Build history of the part. All positions in model axes, mm. A direction names the side the tool comes from. Round coordinates to 2 decimals unless told otherwise and drop trailing zeros. Loops run counter-clockwise (first coordinate to the right, second up) from the corner with the lowest first, then second, coordinate; pieces in that order, holes last. Notation, with made-up numbers: M 71.5,4 L 96.5,4 A9 ccw 96.5,17 Z; hole C 13.5,20 d6. An arc over 180 degrees is marked long. One line per item, written item: value.
```python
from build123d import *

# Parameters (mm, degrees)
F1_W     = 13.4705491364
F1_H     = 26.6246274114
F2_DEPTH = 92.5794709474
F3_W     = 92.5794709474
F3_H     = 21.2339237332
F4_DEPTH = 37.4759007245
F6_DEPTH = 116.4518650621


with BuildPart() as f2:
    # F1 (on face) → F2 (new body)
    with BuildSketch(Plane.XZ):
        Polygon((13.4705491364, 31.8936929107), (13.4705491364, 0), (13.4705491364, -26.6246274114), (13.4705491364, -62.8302171826), (34.1447852552, -62.8302171826), (34.1447852552, 31.8936929107), align=None)
        with Locations((6.7352745682, -13.3123137057)):
            Rectangle(F1_W, F1_H)
        with Locations((-6.7352745682, -13.3123137057)):
            Rectangle(F1_W, F1_H)
        Polygon((-13.4705491364, 0), (-13.4705491364, 31.8936929107), (-34.1447852552, 31.8936929107), (-34.1447852552, -62.8302171826), (-13.4705491364, -62.8302171826), (-13.4705491364, -26.6246274114), align=None)
    extrude(amount=-F2_DEPTH)

    # F3 (on face) → F4 (join)
    with BuildSketch(Plane(origin=(-34.1447852552, 0, 0), x_dir=(0, -1, 0), z_dir=(-1, 0, 0))):
        with Locations((-46.2897354737, -52.213255316)):
            Rectangle(F3_W, F3_H)
    extrude(amount=F4_DEPTH)

    # F5 (on face) → F6 (cut)
    with BuildSketch(Plane.XY.offset(-41.5962934494)):
        Polygon((-71.6206859797, 0), (-34.1447852552, 0), (-71.6206859797, 17.6472961903), align=None)
    extrude(amount=-F6_DEPTH, mode=Mode.SUBTRACT)


solid = f2.part
```
Item 1: Drop flat-ended pins along their axis: P1, Ø4, axis at y = 37, z = -12, coming from the -X side; P2, Ø13.5, axis at x = -6.5, y = 32.5, coming from the +Z side. Give the stop position or say it passes through.
Check values:
P1: stops at x = -34.14
P2: stops at z = 0
Item 2: Pull direction X, two halves, no side cores. Call faces 1 (the face through (24, 46, 31.894)), 2 (the face through (-52.62, 8.7, -52.06)), 3 (the face through (-13.471, 46, 16)), 4 (the face through (34.145, 46, -16)): pulls with the +X half, pulls with the -X half, needs draft (parallel to the pull), parting line crosses it, or undercut.
Check values:
face 1: needs draft
face 2: pulls with the -X half
face 3: undercut
face 4: pulls with the +X half
Item 3: Which spindle directions (+Z, -Z, +X, -X, +Y, -Y) get a long thin tool onto all of the face, cutting with end or side? Do faces 5 (the face through (-34.145, 46, -4)), 6 (the face through (-42, 47, -62.83)), 7 (the face through (13.471, 46, 16)), 8 (the face through (0, 46, -26.625)). Say none if no direction does.
Check values:
face 5: +Z, -X, +Y, -Y
face 6: -Z, +X, -X, +Y, -Y
face 7: +Z, +Y, -Y
face 8: -Z, +Y, -Y
Item 4: Slice it at C-C, the plane y = 77.5. Give the cut face in (x, z), and give its area (3 significant figures).
Check values:
outline: M -71.62,-62.83 L -13.47,-62.83 L -13.47,-26.62 L 13.47,-26.62 L 13.47,-62.83 L 34.14,-62.83 L 34.14,31.89 L 13.47,31.89 L 13.47,0 L -13.47,0 L -13.47,31.89 L -34.14,31.89 L -34.14,-41.6 L -71.62,-41.6 Z
area: 5,430 mm2
Item 5: Slice it at D-D, the plane x = -12. Give the cut face in (y, z), and give its area (3 significant figures).
Check values:
outline: M 0,-26.62 L 92.58,-26.62 L 92.58,0 L 0,0 Z
area: 2,460 mm2
Item 6: Slice it at B-B, the plane z = -49.5. Give the cut face in (x, y).
Check values:
outline: M -71.62,17.65 L -34.14,0 L -13.47,0 L -13.47,92.58 L -71.62,92.58 Z; M 13.47,0 L 34.14,0 L 34.14,92.58 L 13.47,92.58 Z
Item 7: Wall check: line 1 along X through (y, z) = (10.5, 25); line 2 along Z through (x, y) = (-66.5, 48.5); line 3 along Z through (x, y) = (-7, 11). Give the ranges that are in metal, low to high.
Check values:
line 1: x = -34.14 to -13.47, 13.47 to 34.14
line 2: z = -62.83 to -41.6
line 3: z = -26.62 to 0
Item 8: Slice it at A-A, the plane z = 17. Give the cut face in (x, y).
Check values:
outline: M -34.14,0 L -13.47,0 L -13.47,92.58 L -34.14,92.58 Z; M 13.47,0 L 34.14,0 L 34.14,92.58 L 13.47,92.58 Z
